Geometry: see drawing. Coordinates: mm, zero at the bounding-box minimum. A direction names the side the tool comes from. Round coordinates to 2 decimals unless told otherwise and drop trailing zeros. Order: outer loops, then holes, each group sorted by start corner. A loop starts at its lowest first (then second) coordinate and runs counter-clockwise, first axis right, second up. Notation, with made-up numbers: (89.5, 49.5) - (126.5, 49.5) arc R4 ccw to (126.5, 55.5) - close; hole circle Ø8 at (37.5, 64). An arc over 180 degrees is marked (long way). Put each result on its own line as item: value. Start each with the question number.
1) Section A-A on z = 21.5. Output: boundary loops of the cut face in (x, y).
2) Access query for the marked faces 1 and 2. Directions: +Z, -Z, +X, -X, +Y, -Y. A direction counts if a zero-diameter tool reaches every point of the face in a straight line with its end or side. Return the directions, or none.
3) Line query: probe 1 along Z at (x, y) = (14.5, 29); probe 2 along Z at (x, y) = (30.5, 8.5) (1 decimal); probe 3 along Y at (x, z) = (31.5, 9) (1 decimal). Output: solid intervals per line, ascending. Write a range as [from, to].
4) Contact query for flat-ended pins moving along their axis: P1, Ø8, axis at y = 5.5, z = 42, coming from the -X side (1 decimal); P2, Ø8, axis at y = 5, z = 42, coming from the -X side; P3, Ø4, axis at x = 25, y = 23.5, coming from the +Z side. Output: stop coordinate, or through.
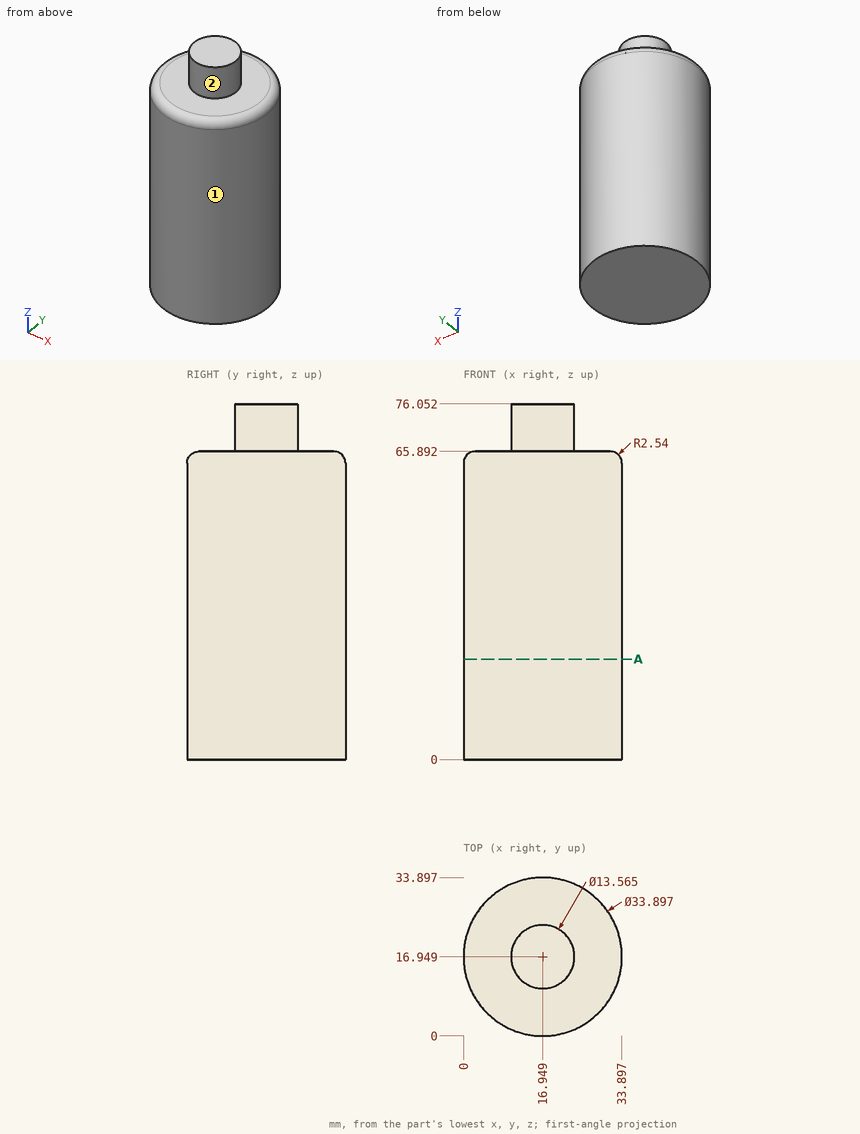
Answer sheet:
1. outline: circle Ø33.9 at (16.95, 16.95)
2. face 1: +Z, -Z
2. face 2: +Z
3. probe 1: [0, 65.89]
3. probe 2: [0, 65.4]
3. probe 3: [8.3, 25.6]
4. P1: x = 1.7
4. P2: x = 1.98
4. P3: z = 65.89
